Design review of the part built by this model. Coordinates are the model's own, in mm. A direction names the side the tool comes from. Coordinates: 2 decimals unless noted, no trailing zeros. Loops run counter-clockwise (first coordinate to the right, second up) from the corner with the lowest first, then second, coordinate; pieces in that order, holes last.
from build123d import *

# Parameters (mm, degrees)
EXTRUDE_1_DEPTH    = 50
SKETCH1_R          = 5
CUT_EXTRUDE1_DEPTH = 20
SKETCH2_W          = 19.36508075
SKETCH2_H          = 147.157362998
CUT_EXTRUDE2_DEPTH = 155.236083451


with BuildPart() as part:
    # Эскиз1 → Вытянуть1 (new body)
    with BuildSketch(Plane.XY):
        Polygon((49.89246994, 41.122656045), (22.824133965, 23.436424123), (22.792974544, -49.563569227), (-22.910878505, -49.563569227), (-22.910878505, 23.436424124), (-49.89246994, 41.122656045), (-49.89246994, 106.450623349), (49.89246994, 106.450623349), align=None)
    extrude(amount=EXTRUDE_1_DEPTH)

    # Sketch1 → Cut-Extrude1 (cut)
    with BuildSketch(Plane.XZ.offset(49.563569227)):
        with Locations(Location((0, 25, 0), (0, 0, 270))):
            Circle(SKETCH1_R)
    extrude(amount=-CUT_EXTRUDE1_DEPTH, mode=Mode.SUBTRACT)

    # Sketch2 → Cut-Extrude2 (cut, through all)
    with BuildSketch(Plane.ZY.offset(49.89246994)):
        with Locations((25, 114.701337544)):
            Rectangle(SKETCH2_W, SKETCH2_H)
    extrude(amount=-CUT_EXTRUDE2_DEPTH, mode=Mode.SUBTRACT)


solid = part.part
Q1. The part is to be moulded in two halves that separate along X. For faces 4 (the flat face through (-1, 106.451, 42)), 5 (the flat face through (49.892, 74, 8)), 6 (the flat face through (0, -29.564, 25)), say which applies: pulls with the +X half, pulls with the -X half, needs draft (parallel to the pull), parting line crosses it, or undercut.
Q2. Take a section at C-C, the plane z = 12. Write out the cut boundary in (x, y), then the cut area to 3 significant figures.
Q3. Take a section at B-B, the plane x = 0. Write out the cut boundary in (y, z).
Q4. Clearance check with flat-ended pins moving along their axes: pin 1 Ø15 at (y, z) = (-8, 19) entering from +X; pin 2 Ø6 at (x, z) = (-32.5, 19) entering from +Y; pin 3 Ø6 at (y, z) = (7.5, 38.5) entering from -X. State where each tip first meets the part, or that it passes through.
Q5. For line 1 (Z direction, x = 5, y = 89); line 2 (X direction, y = -44, z = 25); line 3 (X direction, y = -34.5, z = 45.5), list the stretches that pass through material, from the lowest coordinate up.
Q6. Machinability: for faces 1 (the flat face through (-22.911, -14, 25)), 2 (the flat face through (-1, 73, 15.317)), 3 (the cylindrical face through (0, -40, 30)), which of the approach directions +Z, -Z, +X, -X, +Y, -Y give a long, thin tool a straight path to every point of the face, cutting with its end or side? Answer none if there is none.
Q7. Take a section at D-D, the plane x = -15. Write out the cut boundary in (y, z).
Q8. Take a section at A-A, the plane y = 76.5. Write out the cut boundary in (x, z).
Entries:
1. face 4: needs draft
1. face 5: pulls with the +X half
1. face 6: undercut
2. outline: (-49.89, 41.12) - (-22.91, 23.44) - (-22.91, -49.56) - (22.79, -49.56) - (22.82, 23.44) - (49.89, 41.12) - (49.89, 106.45) - (-49.89, 106.45) - close
2. area: 11,100 mm2
3. outline: (-49.56, 0) - (106.45, 0) - (106.45, 15.32) - (41.12, 15.32) - (41.12, 34.68) - (106.45, 34.68) - (106.45, 50) - (-49.56, 50) - (-49.56, 30) - (-29.56, 30) - (-29.56, 20) - (-49.56, 20) - close
4. pin 1: stops at x = 22.81
4. pin 2: stops at y = 41.12
4. pin 3: stops at x = -22.91
5. line 1: z = 0 to 15.32, 34.68 to 50
5. line 2: x = -22.91 to -5, 5 to 22.8
5. line 3: x = -22.91 to 22.8
6. face 1: +Z, -Z, -X, -Y
6. face 2: +X, -X, +Y
6. face 3: -Y
7. outline: (-49.56, 0) - (106.45, 0) - (106.45, 15.32) - (41.12, 15.32) - (41.12, 34.68) - (106.45, 34.68) - (106.45, 50) - (-49.56, 50) - close
8. outline: (-49.89, 0) - (49.89, 0) - (49.89, 15.32) - (-49.89, 15.32) - close; (-49.89, 34.68) - (49.89, 34.68) - (49.89, 50) - (-49.89, 50) - close
